Can you work these out from the model? Positions are in its coordinate system, mm. A direction names the side the tool comes from. Give positions to 0.01 mm unless a question says otherwise; leave off trailing zeros. Loops run counter-clockwise (first coordinate to the right, second up) from the corner with the lowest first, then second, coordinate; pieces in that order, holes last. Notation, with made-up numbers: (58, -25.5) -> (93, -25.5) arc R3 ccw to (93, -21.5) -> close; hole circle Ø6 at (30, -11). An arc over 180 degrees is marked (long way). Use CSV: the item, a comma, the result in double quotes.
Solid Edge part; units mm, degrees
sketch "Sketch1" plane through (0, 0, 0) normal (1, 0, 0) x (0, 1, 0)
  circle A0 centre (0, 0) radius 20
extrude "Protrusion1" add sketch "Sketch1" along normal mid plane 117
sketch "Sketch2" plane through (-58.5, 0, 0) normal (-1, 0, 0) x (0, -1, 0)
  circle A0 centre (0, 0) radius 20
extrude "ProtrusiónExtruida_2" add sketch "Sketch2" along normal blind 150
sketch "Sketch3" plane through (-74.5, 0, 20) normal (0, 0, 1) x (-1, 0, 0)
  line L0 (-52.5, 6) -> (-96.5, 6)
  arc A0 (-96.5, 6) -> (-102.5, 0) centre (-96.5, 0) ccw
  arc A1 (-102.5, 0) -> (-96.5, -6) centre (-96.5, 0) ccw
  line L1 (-96.5, -6) -> (-52.5, -6)
  arc A2 (-46.5, 0) -> (-52.5, -6) centre (-52.5, 0) cw
  arc A3 (-52.5, 6) -> (-46.5, 0) centre (-52.5, 0) cw
extrude "VaciadoExtruido_3" cut sketch "Sketch3" against normal blind 4.9
chamfer "Chaflán_2" distance 1 angle 45 1 edges at (-208.5, 20, 0)
chamfer "Chaflán_3" distance 1 angle 45 1 edges at (58.5, -20, 0)
sketch "Sketch4" plane through (-208.5, 0, 0) normal (-1, 0, 0) x (0, -1, 0)
  line L0 (-11.449, 16.3988) -> (-10.0101, 14.9599)
  arc A0 (-10.0101, 14.9599) -> (-3.5, 17.6564) centre (0, 0) cw
  line L1 (-3.5, 19.6914) -> (-3.5, 17.6564)
  arc A1 (-11.449, 16.3988) -> (-3.5, 19.6914) centre (0, 0) cw
extrude "VaciadoExtruido_5" cut sketch "Sketch4" against normal blind 30
fillet "Redondeo_3" radius 2 1 edges at (-178.5, 6.8883, 16.6298)
pattern_circular "Pattern1" count 8 over 360 about axis through (-208.5, 0, 0) along (1, 0, 0) of "VaciadoExtruido_5", "Redondeo_3"
(1) We'd pull the mould along Z, two halves only. Please class faces 1 (the face through (-207.99, 13.76, -13.83)), 2 (the face through (-208.5, 0, 0)), 3 (the face through (-194.7, -16.65, 6.84)): released by +Z, released by -Z, zero draft, split by the parting line, or undercut.
Answer sheet:
face 1,"released by -Z"
face 2,"zero draft"
face 3,"undercut"
(2) If we section it at A-A, the plane y = 0: Write out the boundary of the cut face in (x, z), then the cut area to 3 significant figures.
Answer sheet:
outline,"(-208.5, -19) -> (-207.5, -20) -> (57.5, -20) -> (58.5, -19) -> (58.5, 19) -> (57.5, 20) -> (28, 20) -> (28, 15.1) -> (-28, 15.1) -> (-28, 20) -> (-207.5, 20) -> (-208.5, 19) -> close"
area,"10,400 mm2"
(3) Will these pins go through, and if not, where does the flat tip stop? pin 1 Ø6 at (x, y) = (5.5, 1.5) entering from +Z; pin 2 Ø1.6 at (y, z) = (-18, -7.5) entering from -X; pin 3 Ø1 at (x, z) = (-190, 19) entering from +Y; pin 4 Ø2.5 at (y, z) = (7, -17.5) entering from -X.
Answer sheet:
pin 1,"stops at z = 15.1"
pin 2,"stops at x = -178.98"
pin 3,"stops at y = 3.5"
pin 4,"stops at x = -208.5"
(4) If I drill on L1, parallel to Z at x = -161, y = -3.5; L2, parallel to Y at x = -181, z = -7.5; L3, parallel to Y at x = -30, z = 1, over which ranges is the centre line in solid material (lowest first)? Write a range as from..to.
Answer sheet:
L1,"z = -19.69..19.69"
L2,"y = -16.36..16.36"
L3,"y = -19.97..19.97"
(5) Which directions (+Z, -Z, +X, -X, +Y, -Y) give clear straight access to the entire face, cutting with the end or side of a thin tool? Please do faces 4 (the face through (28, 0, 18)), 5 (the face through (-194.696, 6.934, -16.611)), 6 (the face through (-194.7, 6.84, 16.65)), 7 (the face through (-194.7, 16.65, -6.84)).
Answer sheet:
face 4,"+Z"
face 5,"-Z, -X"
face 6,"+Z, -X"
face 7,"-X, +Y"
(6) If we section it at B-B, the plane x = -118: Write out the boundary of the cut face in (y, z), then the cut area to 3 significant figures.
Answer sheet:
outline,"circle Ø40 at (0, 0)"
area,"1,260 mm2"
